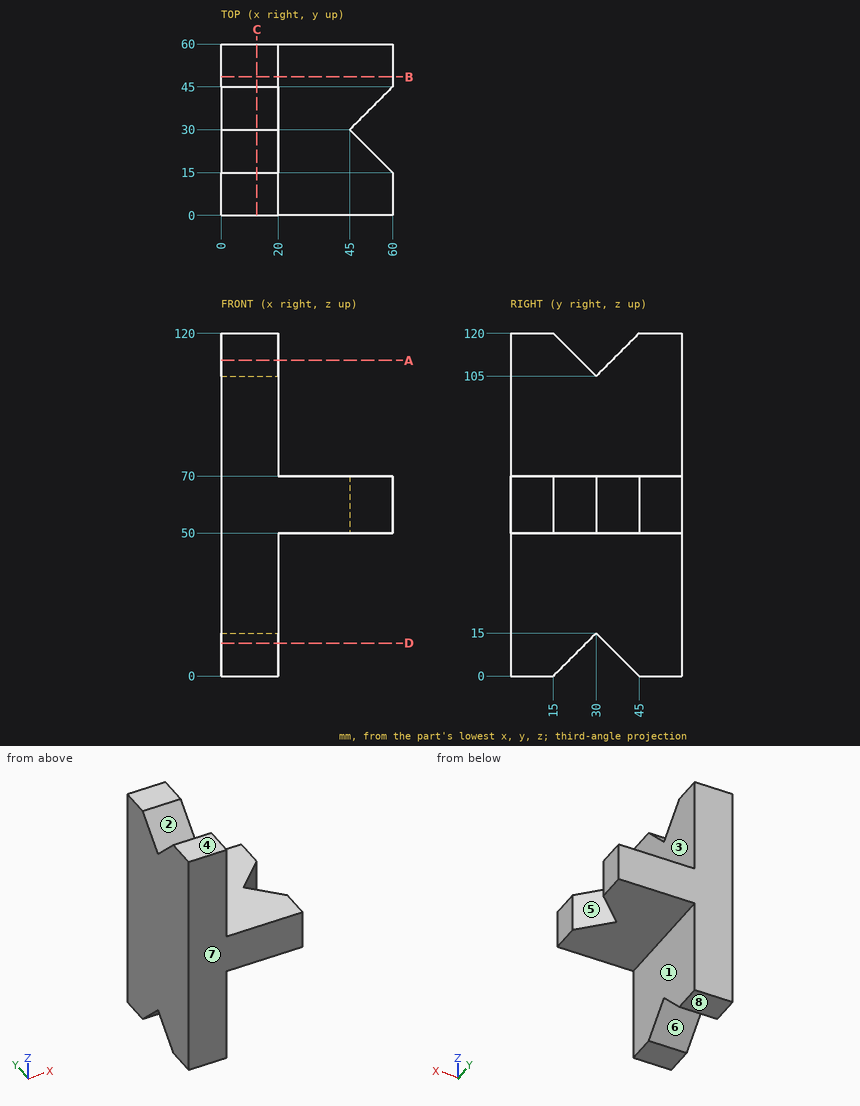
Verification items for this drawing (mm, ordinates from the low corner). A direction names the side the tool comes from. Round coordinates to 2 decimals unless told otherwise and drop trailing zeros. Write each loop counter-clockwise with the first axis right and the second up, starting at its lowest first coordinate (ties: lowest second). Pieces come first, ordered by that corner, then holes. Notation, with made-up numbers: (10.25, -16.75) - (16.25, -16.75) arc R23 cw to (16.25, -1.75) - close; hole circle Ø5 at (-13.75, 27). An arc over 180 degrees is marked (long way). Answer as a JSON object with one key per item and string values. Group by question number.
Q1. Section check D-D, the plane z = 11.5. Enter the section's corners in (x, y).
Q2. Section check B-B, the plane y = 48.5. Enter the section's corners in (x, z), plus the area to 3 significant figures.
Q3. Go/stop test with flat-tipped pins: pin 1 Ø5 at (x, y) = (6.5, 21.5) entering from +Z; pin 2 Ø1 at (x, y) = (30, 46.5) entering from +Z; pin 3 Ø8 at (y, z) = (48, 104.5) entering from +X. Record where each tip stops, or that it passes through.
Q4. Mould release check, pull along Y, two halves, no side actions. Record for the marked faces 6, 7 and 8: released by +Y, released by -Y, zero draft, split by the parting line, or undercut.
Q5. Thickness scan on line 1 (X direction, y = 18, z = 37.5); line 2 (Z direction, x = 21.5, y = 56.5); line 3 (Y direction, x = 8.5, z = 112). Record the ranges inside material, lowest first.
Q6. Tool access check on the marked faces 1, 2, 3, 4 and 5. Record the directions out of +Z, -Z, +X, -X, +Y, -Y that give a thin tool (end or side, any length) a straight path to the whole face; none if there is none.
Q7. Section check A-A, the plane z = 110.5. Enter the section's corners in (x, y).
Q8. Section check C-C, the plane x = 12.5. Enter the section's corners in (y, z), plus the area to 3 significant figures.
Found:
{
 "1": {"outline": "(0, 0) - (20, 0) - (20, 26.5) - (0, 26.5) - close; (0, 33.5) - (20, 33.5) - (20, 60) - (0, 60) - close"},
 "2": {"outline": "(0, 0) - (20, 0) - (20, 50) - (60, 50) - (60, 70) - (20, 70) - (20, 120) - (0, 120) - close", "area": "3,200 mm^2"},
 "3": {"pin 1": "stops at z = 116", "pin 2": "stops at z = 70", "pin 3": "stops at x = 20"},
 "4": {"face 6": "undercut", "face 7": "released by -Y", "face 8": "zero draft"},
 "5": {"line 1": "x = 0 to 20", "line 2": "z = 50 to 70", "line 3": "y = 0 to 23, 37 to 60"},
 "6": {"face 1": "-Z, +X, +Y, -Y", "face 2": "+Z, +X, -X", "face 3": "+Z, +X, +Y, -Y", "face 4": "+Z, +X, -X, +Y, -Y", "face 5": "+Z, -Z, +X"},
 "7": {"outline": "(0, 0) - (20, 0) - (20, 24.5) - (0, 24.5) - close; (0, 35.5) - (20, 35.5) - (20, 60) - (0, 60) - close"},
 "8": {"outline": "(0, 0) - (15, 0) - (30, 15) - (45, 0) - (60, 0) - (60, 120) - (45, 120) - (30, 105) - (15, 120) - (0, 120) - close", "area": "6,750 mm^2"}
}
